Geometry check sheet. Reference: the model listing, model coordinates, mm. Face numbers are marked on the shaded views. A direction names the side the tool comes from. Coordinates: 2 decimals unless noted, no trailing zeros. Write each loop counter-clockwise with the first axis right and the second up, starting at its lowest first coordinate (ties: lowest second). Pieces come first, ordered by that corner, then holes. Notation, with made-up numbers: (-30.75, -33.75) -> (-16.75, -33.75) arc R13 cw to (-16.75, -24.75) -> close; hole circle Ø6 at (-11.5, 48). An arc over 180 degrees is marked (long way). Answer in a Markdown table with one row per item. Add a question column.
Q1. Section check A-A, the plane y = 12. Record the boundary of the cut face in (x, z) (1 decimal), and give its area (3 significant figures).
Q2. Gauge pin test, flat end, axial feed: P1, Ø3.5, axis at x = 0, z = 0, coming from the +Y side. Record the tip position at first contact, or that the pin passes through.
Q3. Thickness scan on line 1 (Z direction, x = 0, y = 7.5) (1 decimal); line 2 (X direction, y = 44, z = 0); line 3 (Y direction, x = -0.25, z = -0.75). Record the ranges inside material, lowest first.
Q4. Section check C-C, the plane y = 29. Record the boundary of the cut face in (x, z) (3 decimals).
Q5. Tool access check on the marked faces 1 and 2. Record the directions out of +Z, -Z, +X, -X, +Y, -Y that give a thin tool (end or side, any length) a straight path to the whole face; none if there is none.
Q6. Release check for a two-part mould opening along X. For the marked faces 3, 4 and 5 record: pulls with the +X half, pulls with the -X half, needs draft (parallel to the pull), parting line crosses it, or undercut.
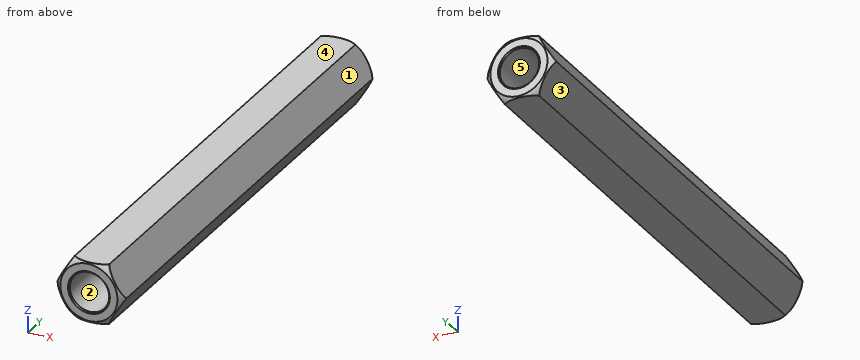
Autodesk Inventor part; units mm, degrees
ref_plane "YZ Plane" through (0, 0, 0) normal (1, 0, 0) x (0, 1, 0)
ref_plane "XZ Plane" through (0, 0, 0) normal (0, 1, 0) x (-1, 0, 0)
ref_plane "XY Plane" through (0, 0, 0) normal (0, 0, 1) x (1, 0, 0)
sketch "Sketch1" plane through (0, 0, 0) normal (0, 1, 0) x (-1, 0, 0)
  line L0 (-1.8331, -3.175) -> (-3.6662, 0)
  line L1 (-3.6662, 0) -> (-1.8331, 3.175)
  line L2 (-1.8331, 3.175) -> (1.8331, 3.175)
  line L3 (1.8331, 3.175) -> (3.6662, 0)
  line L4 (3.6662, 0) -> (1.8331, -3.175)
  line L5 (1.8331, -3.175) -> (-1.8331, -3.175)
  point P0 (0, 0)
  point P1 (0, 0)
  dimension "d0" = 6.35
extrude "Body" add sketch "Sketch1" along normal blind 50.8
sketch "Sketch2" plane through (0, 50.8, 0) normal (0, 1, 0) x (1, 0, 0)
  circle A0 centre (0, 0) radius 2.0955
  dimension "d3" = 4.191
extrude "Hole 2" cut sketch "Sketch2" against normal blind 12.7
sketch "Sketch3" plane through (0, 0, 0) normal (0, -1, 0) x (1, 0, 0)
  circle A0 centre (0, 0) radius 2.0955
  dimension "d6" = 4.191
extrude "Hole 1" cut sketch "Sketch3" against normal blind 12.7
chamfer "Hole 2 Chamfer 1" distance 0.127 distance2 0.1244 1 edges at (-2.0955, 50.8, 0) measured on face at (0.0842, 50.8, 2.8101)
chamfer "Hole 1 Chamfer 1" distance 0.127 distance2 0.1244 1 edges at (-2.0955, 0, 0) measured on face at (-0.0842, 0, 2.8101)
sketch "Sketch4" plane through (0, 0, 0) normal (0, 0, 1) x (1, 0, 0)
  line L0 (1.8331, 50.8) -> (-1.8331, 50.8)
  line L1 (0, 50.8) -> (-3.0353, 50.8)
  line L2 (-3.6662, 50.8) -> (-1.8331, 50.8)
  line L3 (-3.6662, 0) -> (-3.6662, 50.8)
  arc A0 (-3.0353, 50.8) -> (-3.6662, 50.165) centre (-2.2234, 49.3624) ccw
  line L4 (-3.6662, 50.165) -> (-6.3588, 52.7647)
  line L5 (-6.3588, 52.7647) -> (0, 50.8)
  line L6 (0, 50.8) -> (0, 104.464)
  point P0 (0, 0)
  dimension "d15" = 3.0353
  dimension "d16" = 1.651
  dimension "d17" = 0.635
revolve "Hole 2 Chamfer 2" cut sketch "Sketch4" angle 360 about axis through (0, 50.8, 0) along (0, 1, 0)
sketch "Sketch5" plane through (0, 0, 0) normal (0, 0, 1) x (1, 0, 0)
  line L0 (0, 0) -> (-3.0353, 0)
  line L1 (1.8331, 0) -> (-1.8331, 0)
  line L2 (-3.6662, 0) -> (-3.6662, 50.8)
  arc A0 (-3.6662, 0.635) -> (-3.0353, 0) centre (-2.2234, 1.4376) ccw
  line L3 (0, 0) -> (0, -2.1986)
  line L4 (-3.6662, 0.635) -> (-4.1154, -0.8715)
  line L5 (-4.1154, -0.8715) -> (0, 0)
  point P0 (-3.6662, 50.165)
  dimension "d19" = 3.0353
  dimension "d20" = 1.651
  dimension "d21" = 0.635
revolve "Hole 1 Chamfer 2" cut sketch "Sketch5" angle 360 about axis through (0, 0, 0) along (0, -1, 0)
chamfer "Hole 2 Chamfer 1 For Short" [suppressed]
sketch "Sketch7" plane through (0, 0, 0) normal (0, 0, 1) x (1, 0, 0)
  line L0 (0, 50.8004) -> (3.0353, 50.8)
  line L1 (3.6662, 50.8) -> (1.8331, 50.8)
  line L2 (3.6662, 0.635) -> (3.6662, 50.8)
  arc A0 (3.6662, 50.165) -> (3.0353, 50.8) centre (2.2234, 49.3624) ccw
  line L3 (3.6662, 50.165) -> (4.2663, 51.7032)
  line L4 (4.2663, 51.7032) -> (0, 50.8004)
  line L5 (0, 52.6061) -> (0, 50.8004)
  line L6 (1.8331, 50.8) -> (-1.8331, 50.8)
  point P0 (0, 0)
  point P1 (0, 50.8)
  dimension "d33" = 3.0353
  dimension "d34" = 1.651
  dimension "d35" = 0.635
revolve "Hole 2 Chamfer 2 For Short" [suppressed]
properties part number "Standoff .5" material "VEX Aluminum Alloy 5052-H32"
Calculated:
| question | item | result |
|---|---|---|
| 1 | outline | (-3.7, 0) -> (-1.8, -3.2) -> (1.8, -3.2) -> (3.7, 0) -> (1.8, 3.2) -> (-1.8, 3.2) -> close; hole circle Ø4.2 at (0, 0) |
| 1 | area | 21.1 mm² |
| 2 | P1 | stops at y = 38.1 |
| 3 | line 1 | z = -3.2 to -2.1, 2.1 to 3.2 |
| 3 | line 2 | x = -3.67 to -2.1, 2.1 to 3.67 |
| 3 | line 3 | y = 12.7 to 38.1 |
| 4 | outline | (-3.666, 0) -> (-1.833, -3.175) -> (1.833, -3.175) -> (3.666, 0) -> (1.833, 3.175) -> (-1.833, 3.175) -> close |
| 5 | face 1 | +Z, +X, +Y, -Y |
| 5 | face 2 | -Y |
| 6 | face 3 | pulls with the -X half |
| 6 | face 4 | needs draft |
| 6 | face 5 | undercut |
